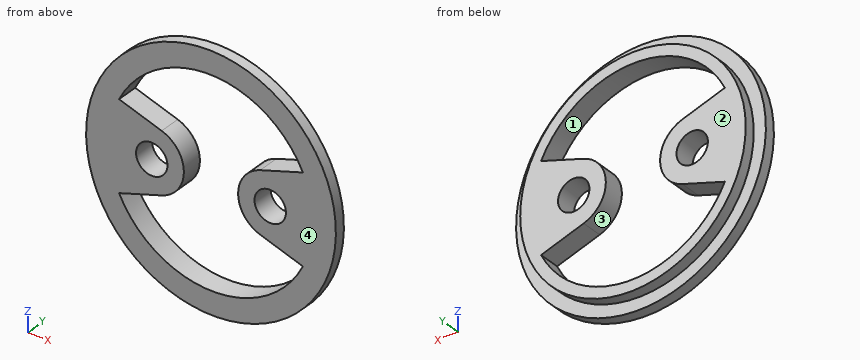
from build123d import *

# Parameters (mm, degrees)
SKETCH2_R           = 17.5
SKETCH2_R_2         = 2.2
BOSS_EXTRUDE2_DEPTH = 3
SKETCH3_OUTSIDE_W   = 46.918
SKETCH3_OUTSIDE_H   = 46.918
SKETCH3_OUTSIDE_R   = 15.8
CUT_EXTRUDE1_DEPTH  = 1.5
CUT_EXTRUDE2_DEPTH  = 25.929901725


with BuildPart() as part:
    # Sketch2 → Boss-Extrude2 (new body)
    with BuildSketch(Plane(origin=(0, 0, 0), x_dir=(1, 0, 0), z_dir=(0, 1, 0))):
        with Locations(Location((0, 0, 0), (0, 0, 270))):
            Circle(SKETCH2_R)
        with Locations(Location((-8.3, 0, 0), (0, 0, 270))):
            Circle(SKETCH2_R_2, mode=Mode.SUBTRACT)
        with Locations(Location((8.3, 0, 0), (0, 0, 90))):
            Circle(SKETCH2_R_2, mode=Mode.SUBTRACT)
    extrude(amount=BOSS_EXTRUDE2_DEPTH)

    # Sketch3 outside → Cut-Extrude1 (cut)
    with BuildSketch(Plane(origin=(0, 3, 0), x_dir=(1, 0, 0), z_dir=(0, 1, 0))):
        Rectangle(SKETCH3_OUTSIDE_W, SKETCH3_OUTSIDE_H)
        with Locations(Location((0, 0, 0), (0, 0, 270))):
            Circle(SKETCH3_OUTSIDE_R, mode=Mode.SUBTRACT)
    extrude(amount=-CUT_EXTRUDE1_DEPTH, mode=Mode.SUBTRACT)

    # Sketch4 → Cut-Extrude2 (cut, through all)
    with BuildSketch(Plane(origin=(0, 3, 0), x_dir=(1, 0, 0), z_dir=(0, 1, 0))):
        with BuildLine():
            ThreePointArc((-6.909423525, 4.279754323), (-3.8, 0), (-6.909423525, -4.279754323))
            Line((-6.909423525, -4.279754323), (-12.877005888, -6.218739372))
            ThreePointArc((-12.877005888, -6.218739372), (0, -14.3), (12.877005888, -6.218739372))
            Line((12.877005888, -6.218739372), (6.909423525, -4.279754323))
            ThreePointArc((6.909423525, -4.279754323), (3.8, 0), (6.909423525, 4.279754323))
            Line((6.909423525, 4.279754323), (12.877005888, 6.218739372))
            ThreePointArc((12.877005888, 6.218739372), (0, 14.3), (-12.877005888, 6.218739372))
            Line((-12.877005888, 6.218739372), (-6.909423525, 4.279754323))
        make_face()
    extrude(amount=-CUT_EXTRUDE2_DEPTH, mode=Mode.SUBTRACT)


solid = part.part
Input: part model. Units: mm. Frame: model coordinates. Face numbers are marked on the shaded views. A direction names the side the tool comes from. Round coordinates to 2 decimals unless told otherwise and drop trailing zeros. Order: outer loops, then holes, each group sorted by start corner. A loop starts at its lowest first (then second) coordinate and runs counter-clockwise, first axis right, second up.
1. Cut plane A-A, the plane z = 0. Output: boundary loops of the cut face in (x, y), then the cut area to 3 significant figures.
The answers:
outline: (-17.5, 0) - (-10.5, 0) - (-10.5, 3) - (-15.8, 3) - (-15.8, 1.5) - (-17.5, 1.5) - close; (-6.1, 0) - (-3.8, 0) - (-3.8, 3) - (-6.1, 3) - close; (3.8, 0) - (6.1, 0) - (6.1, 3) - (3.8, 3) - close; (10.5, 0) - (17.5, 0) - (17.5, 1.5) - (15.8, 1.5) - (15.8, 3) - (10.5, 3) - close
area: 50.7 mm2
2. Cut plane C-C, the plane x = -11. Output: boundary loops of the cut face in (y, z).
The answers:
outline: (0, -13.61) - (1.5, -13.61) - (1.5, -11.34) - (3, -11.34) - (3, -9.14) - (0, -9.14) - close; (0, -5.61) - (3, -5.61) - (3, 5.61) - (0, 5.61) - close; (0, 9.14) - (3, 9.14) - (3, 11.34) - (1.5, 11.34) - (1.5, 13.61) - (0, 13.61) - close
3. Mould query, pull axis Z, two halves, no side actions, for the marked faces 1 and 2. Classes: released by +Z, released by -Z, zero draft, split by the parting line, or undercut.
The answers:
face 1: undercut
face 2: zero draft
4. Set-up query: the marked faces 3 and 4. Return all of +Z, -Z, +X, -X, +Y, -Y with unobstructed straight access to the full face (end or side cutting, diameter ignored); none if empty.
The answers:
face 3: +Y, -Y
face 4: +Z, -Z, +X, -X, -Y
5. Material intervals for line 1 (Z direction, x = -7.5, y = 2.35); line 2 (Z direction, x = 8.3, y = 1.45); line 3 (Z direction, x = 0, y = 0.55), sorted ascending.
The answers:
line 1: z = -13.91 to -12.18, -4.47 to -2.05, 2.05 to 4.47, 12.18 to 13.91
line 2: z = -15.41 to -11.64, -4.73 to -2.2, 2.2 to 4.73, 11.64 to 15.41
line 3: z = -17.5 to -14.3, 14.3 to 17.5
6. Cut plane B-B, the plane y = 2.55. Output: boundary loops of the cut face in (x, z).
The answers:
outline: circle Ø31.6 at (0, 0); hole (-12.88, -6.22) arc R14.3 ccw to (12.88, -6.22) - (6.91, -4.28) arc R4.5 cw to (6.91, 4.28) - (12.88, 6.22) arc R14.3 ccw to (-12.88, 6.22) - (-6.91, 4.28) arc R4.5 cw to (-6.91, -4.28) - close; hole circle Ø4.4 at (-8.3, 0); hole circle Ø4.4 at (8.3, 0)
7. Pin query (flat end, axial travel): P1, Ø5.5, axis at x = -8.3, z = 0, coming from the -Y side; P2, Ø1.5, axis at y = 1, z = 13, coming from the -X side; P3, Ø1, axis at y = 0.5, z = -10.5, coming from the -X side; P4, Ø1.5, axis at x = -3.5, y = 0.5, coming from the +Z side. Return the tip coordinate at first contact, or that it passes through.
The answers:
P1: stops at y = 0
P2: stops at x = -12.5
P3: stops at x = -14.36
P4: stops at z = 17.28
8. Cut plane D-D, the plane z = 9.5. Output: boundary loops of the cut face in (x, y).
The answers:
outline: (-14.7, 0) - (-10.69, 0) - (-10.69, 3) - (-12.62, 3) - (-12.62, 1.5) - (-14.7, 1.5) - close; (10.69, 0) - (14.7, 0) - (14.7, 1.5) - (12.62, 1.5) - (12.62, 3) - (10.69, 3) - close
